Check sheet for the modelled part. Datum: model origin and axes. Units: mm. Give positions to 0.01 mm unless a question says otherwise; leave off trailing zeros. Write each loop counter-clockwise with the first axis right and the second up, starting at its lowest first coordinate (ties: lowest second). Pieces come first, ordered by that corner, then holes. Notation, with made-up numbers: (21.5, 83) -> (70.5, 83) arc R34 cw to (70.5, 114) -> close; hole circle Ø2 at (9.25, -26.5). An arc over 180 degrees is marked (long way). Return JSON: item names as keys, results as strings.
from build123d import *


with BuildPart() as part:
    # Sketch1 → Revolve1 (revolve)
    with BuildSketch(Plane.XY):
        with BuildLine():
            Line((0, 0), (7.5, 0))
            ThreePointArc((7.5, 0), (9.974873734, 1.025126266), (11, 3.5))
            Line((11, 3.5), (11, 31))
            add(Edge.make_bspline(
                [(0, 47), (1.868508868, 47), (0.839979319, 43.098036716), (3.690772078, 40.909332335), (11, 43.731932555), (11, 31)],
                knots=[0, 0, 0, 0, 0.457352926, 0.557352926, 1, 1, 1, 1], degree=3))
            Line((0, 47), (0, 46.7))
            add(Edge.make_bspline(
                [(0, 46.7), (0.089835783, 46.7), (0.286730482, 46.675440139), (0.526826616, 46.561370695), (0.862385089, 46.18251662), (1.044651981, 45.207868135), (1.153282995, 44.076896377), (1.27957898, 43.224881421), (1.526130511, 42.440350235), (2.004678842, 41.769741959), (2.893610253, 41.423589513), (4.086898349, 41.455426541), (5.493916716, 41.46358206), (6.96424187, 41.18629835), (8.123784424, 40.497710935), (8.965606732, 39.51470229), (9.535509298, 38.514305141), (10.020875278, 37.207692702), (10.397250109, 35.559145848), (10.600364695, 33.859238186), (10.685249745, 32.308941091), (10.7, 31.427518579), (10.7, 31)],
                knots=[0, 0, 0, 0, 0.03125, 0.0625, 0.125, 0.25, 0.3125, 0.375, 0.4375, 0.5, 0.5625, 0.625, 0.6875, 0.75, 0.8125, 0.84375, 0.875, 0.90625, 0.9375, 0.96875, 0.984375, 1, 1, 1, 1], degree=3))
            Line((10.7, 31), (10.7, 5.88640066))
            ThreePointArc((10.7, 5.88640066), (9.7627417, 3.62365896), (7.5, 2.68640066))
            Line((7.5, 2.68640066), (0, 2.68640066))
            Line((0, 2.68640066), (0, 0.3))
            Line((0, 0.3), (0, 0))
        make_face()
    revolve(axis=Axis((0, 0, 0), (0, 1, 0)))


solid = part.part
(1) Cross-section at A-A on y = 17.5. Enter the section's corners in (x, z).
Reply:
{"outline": "circle Ø22 at (0, 0); hole circle Ø21.4 at (0, 0)"}
(2) Release check for a two-part mould opening along Y. For faces 1 (the flat face through (0, 2.686, 0)), 2 (the cylindrical face through (-2.38, 17.44, 10.74)), 3 (the flat face through (0, 0, 0)) record: pulls with the +Y half, pulls with the -Y half, needs draft (parallel to the pull), parting line crosses it, or undercut.
Reply:
{"face 1": "undercut", "face 2": "needs draft", "face 3": "pulls with the -Y half"}
(3) Thickness scan on L1, parallel to X at y = 13.5, z = 0; L2, parallel to X at y = 36.5, z = 0.5. Record the ranges inside material, lowest first.
Reply:
{"L1": "-11 to -10.7, 10.7 to 11", "L2": "-10.47 to -10.16, 10.16 to 10.47"}
(4) Depth check by flat-ended pin: pin 1 Ø8 at (x, z) = (3.5, 7) entering from +Y; pin 2 Ø4 at (x, y) = (6.5, 24) entering from +Z; pin 3 Ø2 at (x, y) = (-3, 9) entering from +Z. Enter the tip coordinate at first touch or a pass-through.
Reply:
{"pin 1": "y = 41.75", "pin 2": "z = 10.04", "pin 3": "z = 10.82"}
